```python
from build123d import *

# Parameters (mm, degrees)
BOSS_EXTRUDE1_DEPTH = 2.286
SKETCH3_R           = 2.4638
CUT_EXTRUDE2_DEPTH  = 126.744366856
FILLET1_R           = 2.54


with BuildPart() as part:
    # Sketch1 → Boss-Extrude1 (new body)
    with BuildSketch(Plane(origin=(0, 0, 0), x_dir=(1, 0, 0), z_dir=(0, 1, 0))):
        Polygon((0, 0), (88.9, 0), (88.9, 25.4), (25.4, 25.4), (25.4, 88.9), (0, 88.9), align=None)
    boss_extrude1 = extrude(amount=BOSS_EXTRUDE1_DEPTH)

    # Sketch3 → Cut-Extrude2 (cut, through all)
    with BuildSketch(Plane(origin=(0, 2.286, 0), x_dir=(1, 0, 0), z_dir=(0, 1, 0))):
        with Locations(Location((76.2, 12.7, 0), (0, 0, 270))):
            Circle(SKETCH3_R)
        with Locations(Location((12.7, 12.7, 0), (0, 0, 270))):
            Circle(SKETCH3_R)
        with Locations(Location((12.7, 76.2, 0), (0, 0, 270))):
            Circle(SKETCH3_R)
        with Locations(Location((12.7, 38.1, 0), (0, 0, 270))):
            Circle(SKETCH3_R)
        with Locations(Location((38.1, 12.7, 0), (0, 0, 270))):
            Circle(SKETCH3_R)
    cut_extrude2 = extrude(amount=-CUT_EXTRUDE2_DEPTH, mode=Mode.SUBTRACT)

    # Mirror1: Boss-Extrude1, Cut-Extrude2 across plane
    add(boss_extrude1.mirror(Plane(origin=(0, 2.286, -88.9), x_dir=(0, 0, 1), z_dir=(1, 0, 0))))
    add(cut_extrude2.mirror(Plane(origin=(0, 2.286, -88.9), x_dir=(0, 0, 1), z_dir=(1, 0, 0))), mode=Mode.SUBTRACT)

    # Fillet1
    fillet1_edges = [part.edges().sort_by_distance(p)[0] for p in [
        (25.4, 1.143, -88.9),
        (88.9, 1.143, -25.4),
        (88.9, 1.143, 0),
        (-25.4, 1.143, -88.9),
        (-88.9, 1.143, -25.4),
        (-88.9, 1.143, 0),
    ]]
    fillet(fillet1_edges, radius=FILLET1_R)


solid = part.part
```
Input: part model. Units: mm. Frame: model coordinates. Give positions to 0.01 mm unless a question says otherwise; leave off trailing zeros. Order: outer loops, then holes, each group sorted by start corner. A loop starts at its lowest first (then second) coordinate and runs counter-clockwise, first axis right, second up.
1. Pin query (flat end, axial travel): pin 1 Ø1.1 at (y, z) = (1, -68) entering from +X; pin 2 Ø6.5 at (x, z) = (38.1, -12.7) entering from -Y; pin 3 Ø0.7 at (x, y) = (-51, 0.5) entering from -Z. Return the tip coordinate at first contact, or that it passes through.
Computed:
pin 1: stops at x = 25.4
pin 2: stops at y = 0
pin 3: stops at z = -25.4
2. Draft query along Z for faces 1 (the face through (-40.543, 1.159, -13.021)), 2 (the face through (1, 0, -35)). Return one class per face: released by +Z, released by -Z, zero draft, split by the parting line, or undercut.
Computed:
face 1: undercut
face 2: zero draft
3. Cut plane C-C (z = -76.2). Return loops of the section in (x, y).
Computed:
outline: (-25.4, 0) - (-15.16, 0) - (-15.16, 2.29) - (-25.4, 2.29) - close; (-10.24, 0) - (10.24, 0) - (10.24, 2.29) - (-10.24, 2.29) - close; (15.16, 0) - (25.4, 0) - (25.4, 2.29) - (15.16, 2.29) - close
4. Cut plane B-B (z = -12.7). Return loops of the section in (x, y), and give its area (3 significant figures).
Computed:
outline: (-88.9, 0) - (-78.66, 0) - (-78.66, 2.29) - (-88.9, 2.29) - close; (-73.74, 0) - (-40.56, 0) - (-40.56, 2.29) - (-73.74, 2.29) - close; (-35.64, 0) - (-15.16, 0) - (-15.16, 2.29) - (-35.64, 2.29) - close; (-10.24, 0) - (10.24, 0) - (10.24, 2.29) - (-10.24, 2.29) - close; (15.16, 0) - (35.64, 0) - (35.64, 2.29) - (15.16, 2.29) - close; (40.56, 0) - (73.74, 0) - (73.74, 2.29) - (40.56, 2.29) - close; (78.66, 0) - (88.9, 0) - (88.9, 2.29) - (78.66, 2.29) - close
area: 339 mm2
5. Cut plane D-D (y = 0.7). State how many separate pieces and enclosed holes the cut face has, and give its area (3 significant figures).
Computed:
separate pieces: 1
enclosed holes: 10
area: 7,540 mm2
6. Line query: probe 1 along X at (y, z) = (1.85, -76.2); probe 2 along Z at (x, y) = (-12.7, 1.75); probe 3 along Z at (x, y) = (-38.1, 1.1). Output: solid intervals per line, ascending.
Computed:
probe 1: x = -25.4 to -15.16, -10.24 to 10.24, 15.16 to 25.4
probe 2: z = -88.9 to -78.66, -73.74 to -40.56, -35.64 to -15.16, -10.24 to 0
probe 3: z = -25.4 to -15.16, -10.24 to 0
7. Cut plane A-A (x = -76.2). Return loops of the section in (y, z), and give its area (3 significant figures).
Computed:
outline: (0, -25.4) - (2.29, -25.4) - (2.29, -15.16) - (0, -15.16) - close; (0, -10.24) - (2.29, -10.24) - (2.29, 0) - (0, 0) - close
area: 46.8 mm2
